Autodesk Inventor part; units mm, degrees
ref_plane "YZ Plane" through (0, 0, 0) normal (1, 0, 0) x (0, 1, 0)
ref_plane "XZ Plane" through (0, 0, 0) normal (0, 1, 0) x (-1, 0, 0)
ref_plane "XY Plane" through (0, 0, 0) normal (0, 0, 1) x (1, 0, 0)
sketch "Skizze1" plane through (0, 0, 0) normal (0, 0, 1) x (1, 0, 0)
  circle A0 centre (0, 0) radius 7.5
  circle A1 centre (0, 0) radius 10
  dimension "d0" = 15
  dimension "d1" = 20
extrude "Extrusion1" add sketch "Skizze1" along normal blind 100
sketch "Skizze2" plane through (0, 0, 100) normal (0, 0, 1) x (1, 0, 0)
  circle A0 centre (0, 0) radius 10
extrude "Extrusion2" add sketch "Skizze2" along normal blind 5
chamfer "Fase1" distance 2 angle 45 1 edges at (-10, 0, 105)
properties part number "Magazin"
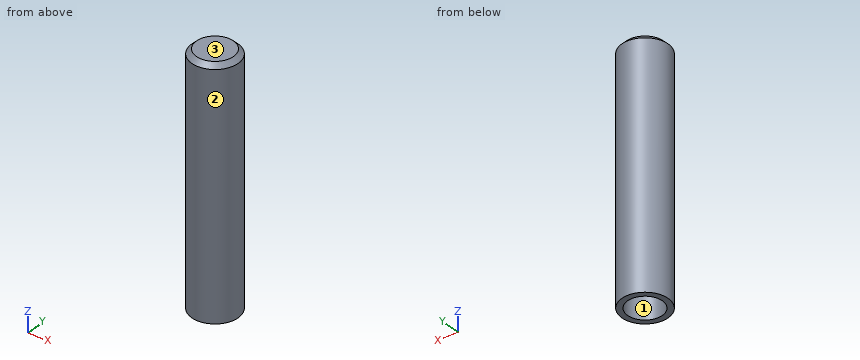
Geometry: final body of the model. Coordinates: model frame, mm. Face numbers are marked on the shaded views. Round coordinates to 2 decimals unless told otherwise and drop trailing zeros. Order: outer loops, then holes, each group sorted by start corner. A loop starts at its lowest first (then second) coordinate and runs counter-clockwise, first axis right, second up. Notation, with made-up numbers: (50, 11) -> (76, 11) arc R21 cw to (76, 45) -> close; hole circle Ø11 at (12.5, 23.25). An arc over 180 degrees is marked (long way). Use one line per item in the form item = value. Start each with the question number.
1. Pin query (flat end, axial travel): pin 1 Ø4 at (x, y) = (-3, -2) entering from -Z; pin 2 Ø1.5 at (x, z) = (-5, 76.5) entering from +Y; pin 3 Ø2 at (x, z) = (1.5, 56.5) entering from +Y. Return the tip coordinate at first contact, or that it passes through.
2. Draft query along X for the marked faces 1, 2 and 3. Return one class per face: pulls with the +X half, pulls with the -X half, needs draft (parallel to the pull), parting line crosses it, or undercut.
3. Cut plane C-C (z = 85.5). Return the cut outline in (x, y), then the cut area to 3 significant figures.
4. Line query: probe 1 along Y at (x, z) = (0, 38.5); probe 2 along Z at (x, y) = (1, 3); probe 3 along Y at (x, z) = (-3.25, 5). Output: solid intervals per line, ascending.
5. Cut plane A-A (y = 0). Return the cut outline in (x, z).
Solution:
q1.pin_1 = 100
q1.pin_2 = 9.05
q1.pin_3 = 9.99
q2.face_1 = undercut
q2.face_2 = parting line crosses it
q2.face_3 = needs draft
q3.outline = circle Ø20 at (0, 0); hole circle Ø15 at (0, 0)
q3.area = 137 mm^2
q4.probe_1 = -10 to -7.5, 7.5 to 10
q4.probe_2 = 100 to 105
q4.probe_3 = -9.46 to -6.76, 6.76 to 9.46
q5.outline = (-10, 0) -> (-7.5, 0) -> (-7.5, 100) -> (7.5, 100) -> (7.5, 0) -> (10, 0) -> (10, 103) -> (8, 105) -> (-8, 105) -> (-10, 103) -> close
